The model under review builds one solid part; all positions refer to its coordinate system, in mm. A direction names the side the tool comes from. Round coordinates to 2 decimals unless told otherwise and drop trailing zeros. Loops run counter-clockwise (first coordinate to the right, second up) from the corner with the lowest first, then second, coordinate; pieces in that order, holes last. Notation, with made-up numbers: M -35,-21.5 L -8,-21.5 A24 ccw -8,1.5 Z; hole C -26.5,23.25 d8. An arc over 180 degrees is marked long. Return JSON: item names as keys, results as strings. Group by question number.
Q1. Clearance check with flat-ended pins moving along their axes: pin 1 Ø6 at (x, z) = (-31, 25) entering from -Y; pin 2 Ø2 at (y, z) = (-8, 3.5) entering from -X; pin 3 Ø2.5 at (x, y) = (47, 27.5) entering from +Z; pin 4 Ø5 at (x, y) = (-46.5, 35) entering from +Z. State where each tip first meets the part, or that it passes through.
Q2. Consider section A-A (y = -0.5). State the section outline as (x, z) points.
Q3. To check wall thickness, follow line 1 along Y through (x, z) = (-52, 13.5); line 2 along X through (y, z) = (-32.5, 28.5); line 3 along Y through (x, z) = (-22.5, 2.15). State the ranges of each line that lie inside material, in increasing order.
Q4. Consider section C-C (y = -28). State the section outline as (x, z) points, and give its area (3 significant figures).
Q5. Draft analysis for pull direction X (two halves, no side actions). For faces 1 (the face through (-1, 1, 0)), 2 (the face through (-45, -48, -5)), 3 (the face through (38.331, 47.535, 10.526)), 4 (the face through (-41.617, -47.465, 34.271)), state which applies: pulls with the +X half, pulls with the -X half, needs draft (parallel to the pull), parting line crosses it, or undercut.
Q6. Consider section B-B (z = 24). Count the separate pieces of the cut face and the enclosed holes in it, and give its area (3 significant figures).
Q7. Consider section D-D (x = 52). State the section outline as (y, z) points, and give its area (3 significant figures).
Q8. For faces 5 (the face through (48, -27, 20)), 6 (the face through (-1, -43, -5)), 7 (the face through (45, 48, -5)), 8 (the face through (47.535, -35.72, 45.504)), list the 3-axis set-ups (+Z, -Z, +X, -X, +Y, -Y) from which the entire face can be reached by the end or side of a thin tool; tool diameter is ignored.
from build123d import *

# Parameters (mm, degrees)
SKETCH_R        = 80
PAD_DEPTH       = 5
PAD001_DEPTH    = 44
SKETCH003_W     = 90
SKETCH003_H     = 90
POCKET_DEPTH    = 44
SKETCH004_R     = 1.75
POCKET001_DEPTH = 49.001
SKETCH005_R     = 17
SKETCH005_R_2   = 60
POCKET002_DEPTH = 5.001
SKETCH006_R     = 16
POCKET003_DEPTH = 119.674913
SKETCH007_R     = 16
POCKET004_DEPTH = 119.674913
SKETCH010_R     = 1.75
POCKET005_DEPTH = 119.674913
PAD002_DEPTH    = 10


with BuildPart() as part:
    # Sketch → Pad (new body)
    with BuildSketch(Plane.XY):
        Circle(SKETCH_R)
    extrude(amount=PAD_DEPTH)

    # Sketch002 → Pad001 (new body)
    with BuildSketch(Plane.XY.offset(5)):
        with BuildLine():
            ThreePointArc((-47.145878, 50), (-55.712311, 55.712311), (-50, 47.145878))
            Line((-50, -47.145878), (-50, 47.145878))
            ThreePointArc((-50, -47.145878), (-55.712311, -55.712311), (-47.145878, -50))
            Line((47.145878, -50), (-47.145878, -50))
            ThreePointArc((47.145878, -50), (55.712311, -55.712311), (50, -47.145878))
            Line((50, 47.145878), (50, -47.145878))
            ThreePointArc((50, 47.145878), (55.712311, 55.712311), (47.145878, 50))
            Line((-47.145878, 50), (47.145878, 50))
        make_face()
    extrude(amount=PAD001_DEPTH)

    # Sketch003 → Pocket (cut)
    with BuildSketch(Plane.XY.offset(49)):
        Rectangle(SKETCH003_W, SKETCH003_H)
    extrude(amount=-POCKET_DEPTH, mode=Mode.SUBTRACT)

    # Sketch004 → Pocket001 (cut, through all)
    with BuildSketch(Plane.XY.offset(49)):
        with Locations((-52, -52)):
            Circle(SKETCH004_R)
        with Locations((52, 52)):
            Circle(SKETCH004_R)
        with Locations((52, -52)):
            Circle(SKETCH004_R)
        with Locations((-52, 52)):
            Circle(SKETCH004_R)
    extrude(amount=-POCKET001_DEPTH, mode=Mode.SUBTRACT)

    # Sketch005 → Pocket002 (cut, through all)
    with BuildSketch(Plane.XY.offset(5)):
        with Locations((-22.5, 22.5)):
            Circle(SKETCH005_R)
        with Locations((22.5, 22.5)):
            Circle(SKETCH005_R)
        with Locations((-22.5, -22.5)):
            Circle(SKETCH005_R)
        with Locations((22.5, -22.5)):
            Circle(SKETCH005_R)
        with Locations((0, -115)):
            Circle(SKETCH005_R_2)
        with Locations((-115, 0)):
            Circle(SKETCH005_R_2)
        with Locations((115, 0)):
            Circle(SKETCH005_R_2)
        with Locations((0, 115)):
            Circle(SKETCH005_R_2)
    extrude(amount=-POCKET002_DEPTH, mode=Mode.SUBTRACT)

    # Sketch006 → Pocket003 (cut, through all)
    with BuildSketch(Plane.YZ.offset(50)):
        with Locations((0, 27)):
            Circle(SKETCH006_R)
        with BuildLine():
            ThreePointArc((-32.145847, 20), (-37.145878, 15.000015), (-32.145878, 10))
            Line((-32.145878, 10), (-22.145878, 10))
            ThreePointArc((-22.145878, 10), (-17.145878, 14.999986), (-22.145849, 20))
            Line((-32.145847, 20), (-22.145849, 20))
        make_face()
        with BuildLine():
            ThreePointArc((22.145861, 20), (17.145878, 14.999992), (22.145878, 10))
            Line((22.145878, 10), (32.145878, 10))
            ThreePointArc((32.145878, 10), (37.145878, 15.000009), (32.14586, 20))
            Line((22.145861, 20), (32.14586, 20))
        make_face()
        with BuildLine():
            ThreePointArc((-32.145895, 54), (-37.145878, 49), (-32.145895, 44))
            Line((-32.145895, 44), (-22.145886, 44))
            ThreePointArc((-22.145886, 44), (-17.145878, 48.999999), (-22.145885, 54))
            Line((-32.145895, 54), (-22.145885, 54))
        make_face()
        with BuildLine():
            ThreePointArc((22.145867, 54), (17.145878, 49), (22.145867, 44))
            Line((22.145867, 44), (32.145858, 44))
            ThreePointArc((32.145858, 44), (37.145878, 49), (32.145857, 54))
            Line((22.145867, 54), (32.145857, 54))
        make_face()
    extrude(amount=-POCKET003_DEPTH, mode=Mode.SUBTRACT)

    # Sketch007 → Pocket004 (cut, through all)
    with BuildSketch(Plane.XZ.offset(50)):
        with Locations((0, 27)):
            Circle(SKETCH007_R)
        with BuildLine():
            ThreePointArc((-32.165386, 54), (-37.165371, 48.999992), (-32.165371, 44))
            Line((-32.165371, 44), (-22.165371, 44))
            ThreePointArc((-22.165371, 44), (-17.165371, 49.000008), (-22.165388, 54))
            Line((-32.165386, 54), (-22.165388, 54))
        make_face()
        with BuildLine():
            ThreePointArc((32.189297, 44), (37.189317, 48.99999), (32.189316, 54))
            Line((32.189316, 54), (22.189316, 54))
            ThreePointArc((22.189316, 54), (17.189317, 49.000008), (22.189299, 44))
            Line((32.189297, 44), (22.189299, 44))
        make_face()
        with BuildLine():
            ThreePointArc((-32.145897, 20), (-37.145878, 14.99999), (-32.145878, 10))
            Line((-32.145878, 10), (-22.145878, 10))
            ThreePointArc((-22.145878, 10), (-17.145878, 15.000011), (-22.145899, 20))
            Line((-32.145897, 20), (-22.145899, 20))
        make_face()
        with BuildLine():
            ThreePointArc((22.145901, 20), (17.145878, 15.000011), (22.145878, 10))
            Line((22.145878, 10), (32.145878, 10))
            ThreePointArc((32.145878, 10), (37.145878, 14.999989), (32.1459, 20))
            Line((22.145901, 20), (32.1459, 20))
        make_face()
    extrude(amount=-POCKET004_DEPTH, mode=Mode.SUBTRACT)

    # Sketch010 → Pocket005 (cut, through all)
    with BuildSketch(Plane(origin=(0, 50, 0), x_dir=(-1, 0, 0), z_dir=(0, 1, 0))):
        with Locations((-40, 34.992924)):
            Circle(SKETCH010_R)
        with Locations((-40, 10)):
            Circle(SKETCH010_R)
        with Locations((40, 10)):
            Circle(SKETCH010_R)
        with Locations((40, 34.941413)):
            Circle(SKETCH010_R)
    extrude(amount=-POCKET005_DEPTH, mode=Mode.SUBTRACT)

    # Sketch008 → Pad002 (new body)
    with BuildSketch(Plane(origin=(0, 0, 0), x_dir=(1, 0, 0), z_dir=(0, 0, -1))):
        with BuildLine():
            ThreePointArc((-40.000017, 53), (-45, 48), (-40.000017, 43))
            Line((-40.000017, 43), (39.999994, 43))
            ThreePointArc((39.999994, 43), (45, 48), (39.999994, 53))
            Line((-40.000017, 53), (39.999994, 53))
        make_face()
        with BuildLine():
            ThreePointArc((-39.99998, -43), (-45, -48), (-39.99998, -53))
            Line((-39.99998, -53), (40.00001, -53))
            ThreePointArc((40.00001, -53), (45, -48), (40.00001, -43))
            Line((-39.99998, -43), (40.00001, -43))
        make_face()
    extrude(amount=PAD002_DEPTH)


solid = part.part
Values:
{
 "1": {"pin 1": "stops at y = -50", "pin 2": "stops at x = -55.68", "pin 3": "stops at z = 44", "pin 4": "stops at z = 49"},
 "2": {"outline": "M -55,0 L 55,0 L 55,5 L 50,5 L 50,11.01 L 45,11.01 L 45,5 L -45,5 L -45,11.01 L -50,11.01 L -50,5 L -55,5 Z; M -50,42.99 L -45,42.99 L -45,49 L -50,49 Z; M 45,42.99 L 50,42.99 L 50,49 L 45,49 Z"},
 "3": {"line 1": "y = -57.25 to -53.75, -50.25 to -46.75, 46.75 to 50.25, 53.75 to 57.25", "line 2": "x = -50 to -45, 45 to 50", "line 3": "y = -59.38 to -39.5, -5.5 to 5.5, 39.5 to 59.38"},
 "4": {"outline": "M -61.93,0 L -38.59,0 L -38.59,5 L -45,5 L -45,10 L -50,10 L -50,5 L -61.93,5 Z; M -50,20 L -45,20 L -45,44 L -50,44 Z; M -6.41,0 L 6.41,0 L 6.41,5 L -6.41,5 Z; M 38.59,0 L 61.93,0 L 61.93,5 L 50,5 L 50,10 L 45,10 L 45,5 L 38.59,5 Z; M 45,20 L 50,20 L 50,44 L 45,44 Z", "area": "588 mm2"},
 "5": {"face 1": "needs draft", "face 2": "pulls with the -X half", "face 3": "undercut", "face 4": "undercut"},
 "6": {"separate pieces": "4", "enclosed holes": "4", "area": "1,560 mm2"},
 "7": {"outline": "M -60.79,0 L -53.75,0 L -53.75,49 L -57.25,49 L -57.25,5 L -60.79,5 Z; M -50.25,0 L 50.25,0 L 50.25,49 L 46.75,49 L 46.75,5 L -46.75,5 L -46.75,49 L -50.25,49 Z; M 53.75,0 L 60.79,0 L 60.79,5 L 57.25,5 L 57.25,49 L 53.75,49 Z", "area": "1,190 mm2"},
 "8": {"face 5": "+X, -X", "face 6": "-Z, +X, -X", "face 7": "-Z, +X", "face 8": "+Z, +X, -X"}
}
